The model under review builds one solid part; all positions refer to its coordinate system, in mm. Face numbers are marked on the shaded views. A direction names the side the tool comes from. Coordinates: 2 decimals unless noted, no trailing zeros. Write each loop counter-clockwise with the first axis right and the second up, starting at its lowest first coordinate (ties: lowest second). Pieces come first, ordered by that corner, then holes.
1) Mouldability with a two-part tool opening along Y and no side actions: class the marked faces 4, 5 and 6 as released by +Y, released by -Y, zero draft, split by the parting line, or undercut.
2) Add section C-C, the plane y = -31. State the section outline as (x, z) points, then the cut area to 3 significant figures.
3) Add section B-B, the plane z = 294. State the section outline as (x, y) points.
4) For line 1 (Z direction, x = 19.5, y = 19); line 2 (Y direction, x = -7, z = 108); line 3 (Z direction, x = 71, y = -155), list the stretches that pass through material, from the lowest coordinate up.
5) Add section A-A, the plane y = 15.5. State the section outline as (x, z) points, then the cut area to 3 significant figures.
6) Machinability: for the marked faces 1, 2 and 3, which of the approach directions +Z, -Z, +X, -X, +Y, -Y give a long, thin tool a straight path to every point of the face, cutting with its end or side? Answer none if there is none.
7) For P1, Ø23.5, axis at x = -50, y = -93.5, coming from the -Z side; P2, Ø4, axis at x = -17.5, z = 263.5, coming from the -Y side; P3, Ø10, axis at y = -53.5, z = 418, coming from the +X side, all flat-tipped, find the tip position at first contact; note any pin that passes through.
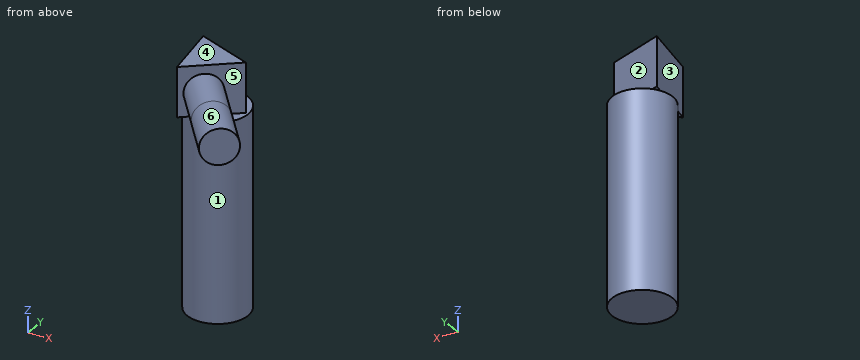
from build123d import *

# Parameters (mm, degrees)
F0_R     = 78.326584
F1_DEPTH = 508
F3_DEPTH = 127
F4_R     = 45.704284
F5_DEPTH = 127
F6_R     = 45.93558
F7_DEPTH = 127


with BuildPart() as f1:
    # F0 (on Top) → F1 (new body)
    with BuildSketch(Plane.XY):
        with Locations((-8.379999, -11.925638)):
            Circle(F0_R)
    extrude(amount=F1_DEPTH)

    # F2 (on face) → F3 (join)
    with BuildSketch(Plane.XY.offset(508)):
        Polygon((-56.977515, -105.344039), (62.533833, -8.963253), (-80.69005, 46.346217), align=None)
    extrude(amount=F3_DEPTH)

    # F4 (on face) → F5 (join)
    with BuildSketch(Plane(origin=(29.023017, -35.988292, 0), x_dir=(0.778411, 0.627755, 0), z_dir=(0.627755, -0.778411, 0))):
        with Locations((-50.197605, 567.723095)):
            Circle(F4_R)
    extrude(amount=F5_DEPTH)

    # F6 (on face) → F7 (join)
    with BuildSketch(Plane(origin=(108.747912, -134.846479, 0), x_dir=(0.778411, 0.627755, 0), z_dir=(0.627755, -0.778411, 0))):
        with Locations((-50.197605, 567.723095)):
            Circle(F6_R)
    extrude(amount=F7_DEPTH)


solid = f1.part
Geometry results:
1. face 4: zero draft
1. face 5: undercut
1. face 6: split by the parting line
2. outline: (-84.35, 0) - (67.59, 0) - (67.59, 508) - (35.21, 508) - (35.21, 635) - (-68.6, 635) - (-68.6, 508) - (-84.35, 508) - close
2. area: 90,400 mm2
3. outline: circle Ø156.65 at (-8.38, -11.93)
4. line 1: z = 0 to 508
4. line 2: y = -90.24 to 66.39
4. line 3: z = 522.75 to 612.69
5. outline: (-81.75, 0) - (64.99, 0) - (64.99, 508) - (-0.81, 508) - (-0.81, 635) - (-75.87, 635) - (-75.87, 508) - (-81.75, 508) - close
5. area: 84,100 mm2
6. face 1: -Z
6. face 2: +Z, +X, +Y
6. face 3: +Z, -X, -Y
7. P1: stops at z = 508
7. P2: stops at y = -89.93
7. P3: stops at x = 60.88
